from build123d import *

# Parameters (mm, degrees)
AUFSATZ_LINEAR_AUSTRAGEN1_DEPTH  = 10
F_10_0_10_DURCHMESSER_BOHRUNG1_D = 10
F_5_0_5_DURCHMESSER_BOHRUNG1_D   = 5
DURCHGANGSLOCH_F_R_M101_D        = 11


with BuildPart() as part:
    # Skizze1 → Aufsatz-Linear austragen1 (new body)
    with BuildSketch(Plane(origin=(0, 0, 0), x_dir=(1, 0, 0), z_dir=(0, 1, 0))):
        with BuildLine():
            Line((-105, 90), (105, 90))
            ThreePointArc((105, 90), (112.071067812, 87.071067812), (115, 80))
            Line((115, 80), (115, 50))
            ThreePointArc((115, 50), (112.071067812, 42.928932188), (105, 40))
            Line((105, 40), (55, 40))
            ThreePointArc((55, 40), (44.393398282, 35.606601718), (40, 25))
            Line((40, 25), (40, -45))
            ThreePointArc((40, -45), (44.393398282, -55.606601718), (55, -60))
            Line((55, -60), (65, -60))
            ThreePointArc((65, -60), (72.071067812, -62.928932188), (75, -70))
            Line((75, -70), (75, -80))
            ThreePointArc((75, -80), (72.071067812, -87.071067812), (65, -90))
            Line((65, -90), (-65, -90))
            ThreePointArc((-65, -90), (-72.071067812, -87.071067812), (-75, -80))
            Line((-75, -80), (-75, -70))
            ThreePointArc((-75, -70), (-72.071067812, -62.928932188), (-65, -60))
            Line((-65, -60), (-55, -60))
            ThreePointArc((-55, -60), (-44.393398282, -55.606601718), (-40, -45))
            Line((-40, -45), (-40, 25))
            ThreePointArc((-40, 25), (-44.393398282, 35.606601718), (-55, 40))
            Line((-55, 40), (-105, 40))
            ThreePointArc((-105, 40), (-112.071067812, 42.928932188), (-115, 50))
            Line((-115, 50), (-115, 80))
            ThreePointArc((-115, 80), (-112.071067812, 87.071067812), (-105, 90))
        make_face()
    extrude(amount=AUFSATZ_LINEAR_AUSTRAGEN1_DEPTH)

    # Ø10.0 (10) Durchmesser Bohrung1 (through all)
    with Locations(Plane(origin=(0, 10, 0), x_dir=(1, 0, 0), z_dir=(0, 1, 0))):
        with Locations((-85, 65), (85, 65)):
            Hole(F_10_0_10_DURCHMESSER_BOHRUNG1_D / 2)

    # Ø5.0 (5) Durchmesser Bohrung1 (through all)
    with Locations(Plane(origin=(0, 0, 0), x_dir=(-1, 0, 0), z_dir=(0, -1, 0))):
        with Locations((77.5, 72.5), (92.5, 57.5), (-92.5, 72.5), (-77.5, 57.5)):
            Hole(F_5_0_5_DURCHMESSER_BOHRUNG1_D / 2)

    # Durchgangsloch für M101 (through all)
    with Locations(Plane(origin=(0, 0, 0), x_dir=(-1, 0, 0), z_dir=(0, -1, 0))):
        with Locations((-25, -5), (-25, -75), (25, -5), (25, -75)):
            Hole(DURCHGANGSLOCH_F_R_M101_D / 2)


solid = part.part
The listing builds one solid part. Answer for the finished solid, in the listing's coordinates (mm). A direction names the side the tool comes from. Coordinates: 2 decimals unless noted, no trailing zeros. Loops run counter-clockwise (first coordinate to the right, second up) from the corner with the lowest first, then second, coordinate; pieces in that order, holes last. Notation, with made-up numbers: M 48,59.25 L 101,59.25 A24 cw 101,83.25 Z; hole C -18.75,62.25 d1. An arc over 180 degrees is marked long. Answer in a Markdown table with one row per item.
1) Given pin 1 (3 mm diameter, centred on y = 3.5, z = 21.5, fed in from +X); pin 2 (6 mm diameter, centred on x = -80, y = 2.5, fed in from +Z); pin 3 (3 mm diameter, centred on y = 6.5, z = 8.5, fed in from -X), each flat-ended and moving along its own axis, determine where each tip first touches the part or whether it passes through.
Answers below:
| item | result |
|---|---|
| pin 1 | x = 40 |
| pin 2 | z = -40 |
| pin 3 | x = -40 |
2) Which of the six approach directions +Z, -Z, +X, -X, +Y, -Y give full straight-line access (tool end or side, diameter ignored) to faces 1 (the flat face through (40, 5, 10)), 2 (the flat face through (-40, 5, 10)), 3 (the flat face through (-75, 5, 75))?
Answers below:
| item | result |
|---|---|
| face 1 | +X, +Y, -Y |
| face 2 | -X, +Y, -Y |
| face 3 | +Z, -X, +Y, -Y |
3) Find the intervals of material crossed by probe 1 along Z at (x, y) = (24.5, 0.75); probe 2 along X at (y, z) = (4.75, 75); probe 3 along Z at (x, y) = (-77.5, 5.75), in increasing order.
Answers below:
| item | result |
|---|---|
| probe 1 | -90 to -0.48, 10.48 to 69.52, 80.48 to 90 |
| probe 2 | -75 to -30.5, -19.5 to 19.5, 30.5 to 75 |
| probe 3 | -90 to -75, -70 to -40 |
4) Find section D-D (x = 46). Determine the outline of the cut face in (y, z).
Answers below:
| item | result |
|---|---|
| outline | M 0,-90 L 10,-90 L 10,-37 L 0,-37 Z; M 0,57 L 10,57 L 10,90 L 0,90 Z |
5) Find section B-B (z = -65). Determine the outline of the cut face in (x, y), then the cut area to 3 significant figures.
Answers below:
| item | result |
|---|---|
| outline | M -115,0 L -90,0 L -90,10 L -115,10 Z; M -80,0 L 80,0 L 80,10 L -80,10 Z; M 90,0 L 115,0 L 115,10 L 90,10 Z |
| area | 2,100 mm^2 |
6) Determine the mould class of faces 4 (the cylindrical face through (71.99, 4.93, 62.85)), 5 (the cylindrical face through (-88, 5, -69)), 6 (the flat face through (-1, 5, -90)) for opening direction X: released by +X, released by -X, zero draft, split by the parting line, or undercut.
Answers below:
| item | result |
|---|---|
| face 4 | released by +X |
| face 5 | undercut |
| face 6 | zero draft |
7) Find section C-C (y = 7.5). Count the separate pieces of the cut face and the enclosed holes in it, then the cut area to 3 significant figures.
Answers below:
| item | result |
|---|---|
| separate pieces | 1 |
| enclosed holes | 10 |
| area | 23,400 mm^2 |
8) Find section A-A (x = -25). Determine the outline of the cut face in (y, z).
Answers below:
| item | result |
|---|---|
| outline | M 0,-90 L 10,-90 L 10,-0.5 L 0,-0.5 Z; M 0,10.5 L 10,10.5 L 10,69.5 L 0,69.5 Z; M 0,80.5 L 10,80.5 L 10,90 L 0,90 Z |
